```python
from build123d import *

# Parameters (mm, degrees)
SKETCH1_R           = 49
BOSS_EXTRUDE1_DEPTH = 16
SKETCH3_R           = 12
BOSS_EXTRUDE2_DEPTH = 25
SKETCH4_R           = 9
CUT_EXTRUDE1_DEPTH  = 42


with BuildPart() as part:
    # Sketch1 → Boss-Extrude1 (new body)
    with BuildSketch(Plane(origin=(0, 0, 0), x_dir=(1, 0, 0), z_dir=(0, 1, 0))):
        Circle(SKETCH1_R)
    extrude(amount=BOSS_EXTRUDE1_DEPTH)

    # Sketch2 → Revolve1 (revolve)
    with BuildSketch(Plane.XY):
        Polygon((-43.5, 22.5), (-40.5, 22.5), (-40.5, 16), (-49, 16), (-49, 17.25), align=None)
    revolve(axis=Axis((0, 16, 0), (0, -1, 0)))

    # Sketch3 → Boss-Extrude2 (add)
    with BuildSketch(Plane.XZ):
        Circle(SKETCH3_R)
    extrude(amount=BOSS_EXTRUDE2_DEPTH)

    # Sketch4 → Cut-Extrude1 (cut, through all)
    with BuildSketch(Plane(origin=(0, 16, 0), x_dir=(1, 0, 0), z_dir=(0, 1, 0))):
        Circle(SKETCH4_R)
    extrude(amount=-CUT_EXTRUDE1_DEPTH, mode=Mode.SUBTRACT)


solid = part.part
```
Source: CAD feature listing. Evaluate the final solid. Frame: model axes, mm. A direction names the side the tool comes from. Give positions to 0.01 mm unless a question says otherwise; leave off trailing zeros. Order: outer loops, then holes, each group sorted by start corner. A loop starts at its lowest first (then second) coordinate and runs counter-clockwise, first axis right, second up. Notation, with made-up numbers: (-27.5, 82.25) -> (-5.5, 82.25) arc R31 ccw to (-5.5, 118.25) -> close; hole circle Ø1 at (-26.75, 6). An arc over 180 degrees is marked (long way). Use a Markdown table: item, result.
Q1. Section B-B (z = 0). Return the cut outline in (x, y).
A:
| item | result |
|---|---|
| outline | (-49, 0) -> (-12, 0) -> (-12, -25) -> (-9, -25) -> (-9, 16) -> (-40.5, 16) -> (-40.5, 22.5) -> (-43.5, 22.5) -> (-49, 17.25) -> close; (9, -25) -> (12, -25) -> (12, 0) -> (49, 0) -> (49, 17.25) -> (43.5, 22.5) -> (40.5, 22.5) -> (40.5, 16) -> (9, 16) -> close |
Q2. Section A-A (x = 0). Return the cut outline in (y, z), and give its area (3 significant figures).
A:
| item | result |
|---|---|
| outline | (-25, -12) -> (0, -12) -> (0, -49) -> (17.25, -49) -> (22.5, -43.5) -> (22.5, -40.5) -> (16, -40.5) -> (16, -9) -> (-25, -9) -> close; (-25, 9) -> (16, 9) -> (16, 40.5) -> (22.5, 40.5) -> (22.5, 43.5) -> (17.25, 49) -> (0, 49) -> (0, 12) -> (-25, 12) -> close |
| area | 1,510 mm^2 |
Q3. Section C-C (y = -5). Return the cut outline in (x, z), and give its area (3 significant figures).
A:
| item | result |
|---|---|
| outline | circle Ø24 at (0, 0); hole circle Ø18 at (0, 0) |
| area | 198 mm^2 |
Q4. First-contact query: P1, Ø12, axis at y = -14, z = 1, coming from the -X side; P2, Ø10, axis at x = -4.5, y = 10, coming from the +Z side; P3, Ø2, axis at x = 20.5, y = 7, coming from the +Z side. Flat tips, straight axial feed; report the tip coordinate or a pass-through.
A:
| item | result |
|---|---|
| P1 | x = -12 |
| P2 | z = 49 |
| P3 | z = 44.95 |
Q5. Pull-direction query (Z, two-part tool) for faces 1 (the face through (-1.172, -4.213, -8.923)), 2 (the face through (10, 0, 10)), 3 (the face through (9.488, 22.245, 42.726)); classes: +Z half, -Z half, draft (parallel to the pull), parting line (faces both ways), or undercut.
A:
| item | result |
|---|---|
| face 1 | undercut |
| face 2 | draft |
| face 3 | parting line |
Q6. Material intervals for line 1 (Z direction, x = 0.5, y = -17.5); line 2 (Y direction, x = 16.5, z = 35.5); line 3 (X direction, y = 18.25, z = 0), sorted ascending. Write a range as [from, to].
A:
| item | result |
|---|---|
| line 1 | [-11.99, -8.99], [8.99, 11.99] |
| line 2 | [0, 16] |
| line 3 | [-47.95, -40.5], [40.5, 47.95] |
Q7. Access query for faces 4 (the face through (2, -25, 9)), 5 (the face through (-1, 16, -10)), 6 (the face through (-11.99, -12.32, 0.53)). Directions: +Z, -Z, +X, -X, +Y, -Y. A direction counts if a zero-diameter tool reaches every point of the face in a straight line with its end or side. Return the directions, or none.
A:
| item | result |
|---|---|
| face 4 | +Z, -Z, +X, -X, -Y |
| face 5 | +Y |
| face 6 | -Y |
